from build123d import *

# Parameters (mm, degrees)
SKETCH1_W           = 64
SKETCH1_H           = 67
BOSS_EXTRUDE1_DEPTH = 19
SKETCH2_W           = 8
SKETCH2_H           = 4
BOSS_EXTRUDE2_DEPTH = 1.5
FILLET1_R           = 2


with BuildPart() as part:
    # Sketch1 → Boss-Extrude1 (new body)
    with BuildSketch(Plane.XY):
        Rectangle(SKETCH1_W, SKETCH1_H)
    extrude(amount=BOSS_EXTRUDE1_DEPTH)

    # Sketch2 → Boss-Extrude2 (add)
    with BuildSketch(Plane.XY.offset(19)):
        with Locations((21, 27.5)):
            Rectangle(SKETCH2_W, SKETCH2_H)
    extrude(amount=BOSS_EXTRUDE2_DEPTH)

    # Fillet1
    fillet1_edges = [part.edges().sort_by_distance(p)[0] for p in [
        (32, 0, 19),
        (-32, 0, 19),
        (32, 0, 0),
        (-32, 0, 0),
    ]]
    fillet(fillet1_edges, radius=FILLET1_R)


solid = part.part
Work out the finished part from the listing and answer in its coordinate system (mm). A direction names the side the tool comes from. Coordinates: 2 decimals unless noted, no trailing zeros. Write each loop counter-clockwise with the first axis right and the second up, starting at its lowest first coordinate (ties: lowest second). Pieces come first, ordered by that corner, then holes. Notation, with made-up numbers: M 37,-32.5 L 82,-32.5 A23 ccw 82,-10.5 Z; hole C -3.75,18.5 d11. An arc over 180 degrees is marked long. Answer as CSV lines item,"result". Start each with the question number.
Item 1: A tool of negligible diameter and unlimited length cuts with its end or side. For faces 1 (the face through (-31.43, 0.47, 0.6)), 2 (the face through (17, 27, 20)), 3 (the face through (21, 29.5, 20)), 4 (the face through (21, 25.5, 20)), 5 (the face through (25, 27, 20)), from which of +Z, -Z, +X, -X, +Y, -Y can it reach the whole face along a straight path? Write none if from no direction.
Item 2: Consider L1, parallel to Z at x = 20, y = 24; L2, parallel to X at y = -8, z = 1; L3, parallel to X at y = -5.5, z = 1.5. Determine where each line is inside the solid, lowest interval first.
Item 3: Section A-A on y = -0.5 is taken. Write down the section's boundary in (x, z), and give its area (3 significant figures).
Item 4: Flat-ended cylindrical pins translate along their axes: P1, Ø1.2, axis at x = 21, z = 20, coming from the +Y side; P2, Ø2, axis at x = -3.5, y = -7.5, coming from the +Z side; P3, Ø0.8, axis at y = 28.5, z = 19.5, coming from the -X side. Find the tip coordinate at first contact, or state that the pin passes through.
Item 5: Section B-B on x = -17 is taken. Write down the section's boundary in (y, z).
Checks:
1,face 1,"-Z, -X, +Y, -Y"
1,face 2,"+Z, -X, +Y, -Y"
1,face 3,"+Z, +X, -X, +Y"
1,face 4,"+Z, +X, -X, -Y"
1,face 5,"+Z, +X, +Y, -Y"
2,L1,"z = 0 to 19"
2,L2,"x = -31.73 to 31.73"
2,L3,"x = -31.94 to 31.94"
3,outline,"M -32,2 A2 ccw -30,0 L 30,0 A2 ccw 32,2 L 32,17 A2 ccw 30,19 L -30,19 A2 ccw -32,17 Z"
3,area,"1,210 mm²"
4,P1,"stops at y = 29.5"
4,P2,"stops at z = 19"
4,P3,"stops at x = 17"
5,outline,"M -33.5,0 L 33.5,0 L 33.5,19 L -33.5,19 Z"
